```python
from build123d import *

# Parameters (mm, degrees)
ESTRUSIONE_ESTRUSIONE1_DEPTH = 100
SCHIZZO2_W                   = 100
SCHIZZO2_H                   = 100
SCHIZZO2_W_2                 = 90
SCHIZZO2_H_2                 = 90
ESTRUSIONE_ESTRUSIONE2_DEPTH = 2500
SCHIZZO3_W                   = 100
SCHIZZO3_H                   = 100
ESTRUSIONE_ESTRUSIONE3_DEPTH = 5


with BuildPart() as part:
    # Schizzo1 → Estrusione-Estrusione1 (new body, symmetric)
    with BuildSketch(Plane.XY):
        Polygon((0, 0), (100, 0), (100, 50), (-100, 50), (-100, 0), align=None)
    extrude(amount=ESTRUSIONE_ESTRUSIONE1_DEPTH, both=True)

    # Schizzo2 → Estrusione-Estrusione2 (add)
    with BuildSketch(Plane(origin=(0, 50, 0), x_dir=(1, 0, 0), z_dir=(0, 1, 0))):
        Rectangle(SCHIZZO2_W, SCHIZZO2_H)
        with Locations((-0.272675023, -0.401025499)):
            Rectangle(SCHIZZO2_W_2, SCHIZZO2_H_2, mode=Mode.SUBTRACT)
    extrude(amount=ESTRUSIONE_ESTRUSIONE2_DEPTH)

    # Schizzo3 → Estrusione-Estrusione3 (add)
    with BuildSketch(Plane(origin=(0, 2550, 0), x_dir=(1, 0, 0), z_dir=(0, 1, 0))):
        Rectangle(SCHIZZO3_W, SCHIZZO3_H)
    extrude(amount=ESTRUSIONE_ESTRUSIONE3_DEPTH)


solid = part.part
```
Here's how the part is built. I have some questions about the finished solid (model axes, mm). A direction names the side the tool comes from. Give positions to 0.01 mm unless a question says otherwise; leave off trailing zeros. Order: outer loops, then holes, each group sorted by start corner. A loop starts at its lowest first (then second) coordinate and runs counter-clockwise, first axis right, second up. Notation, with made-up numbers: (67, 31) - (112, 31) arc R26 cw to (112, 58) - close; hole circle Ø9 at (83, 58). An arc over 180 degrees is marked (long way). Answer as a JSON object with one key per item and string values. Group by question number.
Item 1: If we section it at B-B on x = 13.5: Please give me the cut outline in (y, z).
Item 2: Which directions (+Z, -Z, +X, -X, +Y, -Y) give clear straight access to the entire face, cutting with the end or side of a thin tool? Please do faces 5 (the flat face through (-1, 1285, -50)), 6 (the flat face through (-45.273, 1282, 1)), 7 (the flat face through (-1, 1285, 50)), 8 (the flat face through (50, 1285, 1)), 9 (the flat face through (-50, 1285, 1)).
Item 3: Please list where these lines run through material, in increasing order: probe 1 along X at (y, z) = (170, 38.5); probe 2 along Y at (x, z) = (-8, 11); probe 3 along Z at (x, y) = (-25, 1100.5).
Item 4: For P1, Ø1, axis at x = 27.5, y = 1649, coming from the +Z side; P2, Ø8, axis at y = 1753.5, z = 38, coming from the +X side; P3, Ø6, axis at y = 1051, z = 47.5, coming from the -X side, each with a flat end and sliding along its axis, tell me the tip position at first contact or that it passes through.
Item 5: If we mould it in two halves opening along X, with no side actions, what happens to faces 1 (the flat face through (-1, 25, -100)), 2 (the flat face through (100, 25, 1)), 3 (the flat face through (-1, 1282, -44.599)), 4 (the flat face through (-1, 1282, 45.401))? For each: pulls with the +X half, pulls with the -X half, needs draft (parallel to the pull), parting line crosses it, or undercut.
Item 6: If we section it at A-A on z = -19: Please give me the cut outline in (x, y).
Item 7: If we section it at C-C on y = 1295.5: Please give me the cut outline in (x, z).
Result set:
{
 "1": {"outline": "(0, -100) - (50, -100) - (50, -50) - (2555, -50) - (2555, 50) - (50, 50) - (50, 100) - (0, 100) - close; hole (50, -44.6) - (2550, -44.6) - (2550, 45.4) - (50, 45.4) - close"},
 "2": {"face 5": "-Z, +X, -X, +Y", "face 6": "none", "face 7": "+Z, +X, -X, +Y", "face 8": "+Z, -Z, +X, +Y", "face 9": "+Z, -Z, -X, +Y"},
 "3": {"probe 1": "-50 to -45.27, 44.73 to 50", "probe 2": "0 to 50, 2550 to 2555", "probe 3": "-50 to -44.6, 45.4 to 50"},
 "4": {"P1": "z = 50", "P2": "x = 50", "P3": "x = -50"},
 "5": {"face 1": "needs draft", "face 2": "pulls with the +X half", "face 3": "undercut", "face 4": "undercut"},
 "6": {"outline": "(-100, 0) - (100, 0) - (100, 50) - (50, 50) - (50, 2555) - (-50, 2555) - (-50, 50) - (-100, 50) - close; hole (-45.27, 50) - (44.73, 50) - (44.73, 2550) - (-45.27, 2550) - close"},
 "7": {"outline": "(-50, -50) - (50, -50) - (50, 50) - (-50, 50) - close; hole (-45.27, -44.6) - (44.73, -44.6) - (44.73, 45.4) - (-45.27, 45.4) - close"}
}
